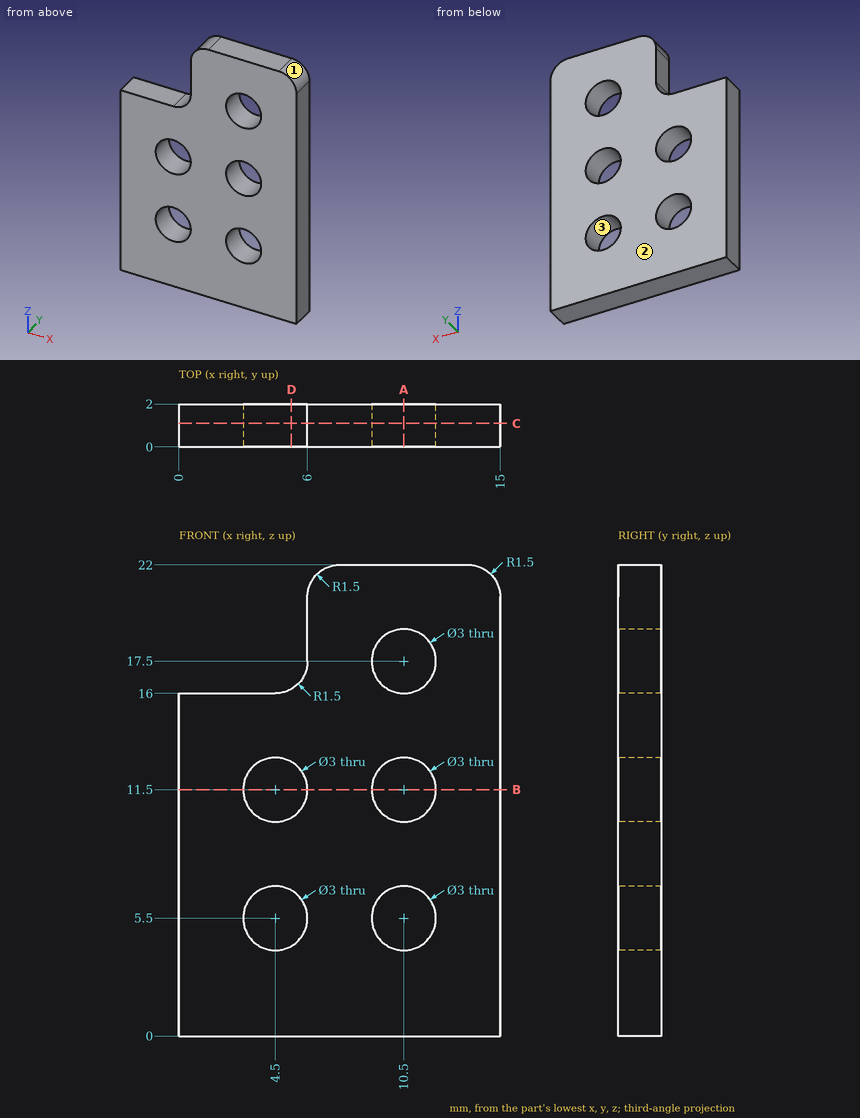
Here's the drawing with two shaded views (mm, measured from the low corner). I have some questions. Give positions to 0.01 mm unless a question says otherwise; leave off trailing zeros. Loops run counter-clockwise (first coordinate to the right, second up) from the corner with the lowest first, then second, coordinate; pieces in that order, holes last. Notation, with made-up numbers: M 71.25,16.25 L 113.25,16.25 A10 ccw 113.25,31.25 Z; hole C -33,-27.5 d3. An arc over 180 degrees is marked long. One line per item, written item: value.
(1) Suppose I cut it at A-A on x = 10.5. List the corners of the cut face in (y, z) for me, plus the area to 3 significant figures.
Returned:
outline: M 0,0 L 2,0 L 2,4 L 0,4 Z; M 0,7 L 2,7 L 2,10 L 0,10 Z; M 0,13 L 2,13 L 2,16 L 0,16 Z; M 0,19 L 2,19 L 2,22 L 0,22 Z
area: 26.0 mm^2
(2) I need wall thicknesses on line 1 (Z direction, x = 4.5, y = 1.4); line 2 (Z direction, x = 10.5, y = 1.8); line 3 (X direction, y = 1.9, z = 12.5). Which ranges of each line are inside material? Lowest first, please.
Returned:
line 1: 0 to 4, 7 to 10, 13 to 16
line 2: 0 to 4, 7 to 10, 13 to 16, 19 to 22
line 3: 0 to 3.38, 5.62 to 9.38, 11.62 to 15
(3) Suppose I cut it at B-B on z = 11.5. List the corners of the cut face in (x, y) for me, plus the area to 3 significant figures.
Returned:
outline: M 0,0 L 3,0 L 3,2 L 0,2 Z; M 6,0 L 9,0 L 9,2 L 6,2 Z; M 12,0 L 15,0 L 15,2 L 12,2 Z
area: 18.0 mm^2
(4) Suppose I cut it at C-C on y = 1.1. List the corners of the cut face in (x, z) for me.
Returned:
outline: M 0,0 L 15,0 L 15,20.5 A1.5 ccw 13.5,22 L 7.5,22 A1.5 ccw 6,20.5 L 6,17.5 A1.5 cw 4.5,16 L 0,16 Z; hole C 4.5,5.5 d3; hole C 4.5,11.5 d3; hole C 10.5,5.5 d3; hole C 10.5,11.5 d3; hole C 10.5,17.5 d3
(5) Suppose I cut it at D-D on x = 5.25. List the corners of the cut face in (y, z) for me.
Returned:
outline: M 0,0 L 2,0 L 2,4.2 L 0,4.2 Z; M 0,6.8 L 2,6.8 L 2,10.2 L 0,10.2 Z; M 0,12.8 L 2,12.8 L 2,16.2 L 0,16.2 Z
(6) We'd pull the mould along Z, two halves only. Please class the marked faces 1, 2 and 3: released by +Z, released by -Z, zero draft, split by the parting line, or undercut.
Returned:
face 1: released by +Z
face 2: zero draft
face 3: undercut
(7) Will this pin go through, and if not, where does the flat tip stop? pin 1 (0.6 mm diameter, centred on x = 3, y = 0.5, fed in from +Z).
Returned:
pin 1: z = 16
